Read the model definition and answer for the solid it produces. Units are mm, in the model's axes. Face numbers are marked on the shaded views. Round coordinates to 2 decimals unless told otherwise and drop trailing zeros. Write each loop counter-clockwise with the first axis right and the second up, starting at its lowest first coordinate (ties: lowest second). Pieces come first, ordered by that corner, then holes. Notation, with made-up numbers: (24, -15) -> (53, -15) arc R15 cw to (53, 1) -> close; hole circle Ø8 at (59.25, 41). An arc over 180 degrees is marked (long way). Return JSON: item names as keys, results as strings.
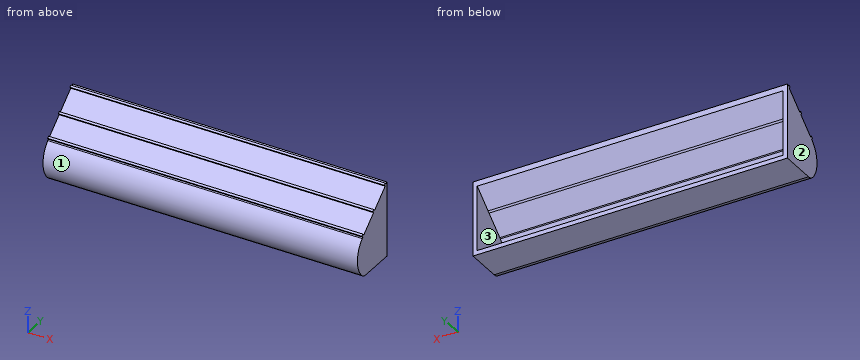
from build123d import *

# Parameters (mm, degrees)
F1_DEPTH    = 55.5
F2_DEPTH    = 297.5
F3_T        = 4
F3_T3_DEPTH = 305.5
F4_R        = 9
F5_R        = 9


# Not quite as in the source:
# - a shell that OpenCascade refuses in one call is made with other operations: the cavity is built on its own and cut out
# - a feature names something its author has since deleted; it is built from what else it names


with BuildPart() as f1:
    # F0 (on Right) → F1 (new body)
    with BuildSketch(Plane.YZ):
        with BuildLine():
            Line((-572.7275457045, -8.2819332473), (-535.7275457045, -8.2819332473))
            Line((-535.7275457045, -8.2819332473), (-535.7275457045, 62.5302098664))
            Line((-535.7275457045, 62.5302098664), (-537.1212494235, 61.363881769))
            Line((-537.1212494235, 61.363881769), (-538.6550321213, 60.0803278606))
            Line((-538.6550321213, 60.0803278606), (-555.619452014, 45.8835661626))
            Line((-555.619452014, 45.8835661626), (-557.1532347119, 44.6000122542))
            Line((-557.1532347119, 44.6000122542), (-572.8000965488, 31.5058557652))
            Line((-572.8000965488, 31.5058557652), (-574.3338792466, 30.2223018568))
            Line((-574.3338792466, 30.2223018568), (-575.2947741996, 29.4181719927))
            ThreePointArc((-575.2947741996, 29.4181719927), (-582.8883712939, 9.9636162879), (-572.7275457045, -8.2819332473))
        make_face()
        Polygon((-538.6550321213, 60.0803278606), (-537.1212494235, 61.363881769), (-538.404803332, 62.8976644668), (-539.9385860298, 61.6141105584), align=None)
        Polygon((-575.6174331551, 31.7560845546), (-574.3338792466, 30.2223018568), (-572.8000965488, 31.5058557652), (-574.0836504573, 33.0396384631), align=None)
        Polygon((-557.1532347119, 44.6000122542), (-555.619452014, 45.8835661626), (-556.9030059225, 47.4173488605), (-558.4367886203, 46.133794952), align=None)
    extrude(amount=F1_DEPTH)

    # F0 (on Right) → F2 (join)
    with BuildSketch(Plane.YZ):
        with BuildLine():
            Line((-572.7275457045, -8.2819332473), (-535.7275457045, -8.2819332473))
            Line((-535.7275457045, -8.2819332473), (-535.7275457045, 62.5302098664))
            Line((-535.7275457045, 62.5302098664), (-537.1212494235, 61.363881769))
            Line((-537.1212494235, 61.363881769), (-538.6550321213, 60.0803278606))
            Line((-538.6550321213, 60.0803278606), (-555.619452014, 45.8835661626))
            Line((-555.619452014, 45.8835661626), (-557.1532347119, 44.6000122542))
            Line((-557.1532347119, 44.6000122542), (-572.8000965488, 31.5058557652))
            Line((-572.8000965488, 31.5058557652), (-574.3338792466, 30.2223018568))
            Line((-574.3338792466, 30.2223018568), (-575.2947741996, 29.4181719927))
            ThreePointArc((-575.2947741996, 29.4181719927), (-582.8883712939, 9.9636162879), (-572.7275457045, -8.2819332473))
        make_face()
        Polygon((-538.6550321213, 60.0803278606), (-537.1212494235, 61.363881769), (-538.404803332, 62.8976644668), (-539.9385860298, 61.6141105584), align=None)
        Polygon((-575.6174331551, 31.7560845546), (-574.3338792466, 30.2223018568), (-572.8000965488, 31.5058557652), (-574.0836504573, 33.0396384631), align=None)
        Polygon((-557.1532347119, 44.6000122542), (-555.619452014, 45.8835661626), (-556.9030059225, 47.4173488605), (-558.4367886203, 46.133794952), align=None)
    extrude(amount=F2_DEPTH)

    # F3: shell of thickness 4, made by hand


with BuildPart() as f3_core1:
    # F3_t2: copy of F1
    add(f1.part)

    # the walls: a layer under each face that stays
    f3_faces = [f3_core1.faces().sort_by_distance(p)[0] for p in [
        (148.75, -582.8883712939, 9.9636162879),
        (0, -559.3362720247, 27.3078656098),
        (148.75, -574.9756562009, 30.9891932057),
        (148.75, -574.8505418062, 32.3978615088),
        (148.75, -573.441873503, 32.2727471141),
        (148.75, -564.9766656303, 38.0529340097),
        (148.75, -557.7950116661, 45.3669036031),
        (148.75, -557.6698972714, 46.7755719063),
        (148.75, -556.2612289683, 46.6504575116),
        (148.75, -547.1372420677, 52.9819470116),
        (148.75, -539.2968090756, 60.8472192095),
        (148.75, -539.1716946809, 62.2558875126),
        (148.75, -537.7630263777, 62.1307731179),
        (148.75, -536.424397564, 61.9470458177),
        (148.75, -554.2275457045, -8.2819332473),
        (297.5, -559.3362720247, 27.3078656098),
        (148.75, -574.8143267231, 29.8202369247),
    ]]
    thicken(f3_faces, amount=-F3_T, mode=Mode.SUBTRACT)

    # F3_s4 → F3_t3 (cut)
    with BuildSketch(Plane.YZ.offset(-4)):
        Polygon((-574.3902259788, 30.2273064326), (-571.266313851, 32.7894096737), (-568.6992060341, 29.721844278), (-571.7667714298, 27.1547364611), align=None)
        Polygon((-572.795091973, 31.5622024973), (-575.8676619445, 28.9387479484), (-573.3005541276, 25.8711825527), (-570.232988732, 28.4382903696), align=None)
        Polygon((-557.209581444, 44.60501683), (-554.586126895, 41.5324468586), (-551.5185614994, 44.0995546754), (-554.0856693162, 47.1671200711), align=None)
        Polygon((-555.6144474383, 45.9399128948), (-558.6870174097, 43.3164583458), (-556.1199095928, 40.2488929501), (-553.0523441972, 42.816000767), align=None)
        Polygon((-538.7113788535, 60.0853324364), (-536.0879243045, 57.0127624649), (-533.0203589088, 59.5798702818), (-535.5874667257, 62.6474356775), align=None)
        Polygon((-537.1162448477, 61.4202285011), (-540.1888148192, 58.7967739522), (-537.6217070023, 55.7292085565), (-534.5541416067, 58.2963163734), align=None)
    extrude(amount=F3_T3_DEPTH, mode=Mode.SUBTRACT)


with BuildPart() as f1_1:
    add(f1.part)

    # what is left inside the walls is the cavity
    f3_cavity = [f3_core1.part.solids().sort_by_distance(p)[0] for p in [
        (197, -535.767546, 26.516207),
    ]]
    add(f3_cavity, mode=Mode.SUBTRACT)

    # F4
    f4_edges = [f1_1.edges().sort_by_distance(p)[0] for p in [
        (148.75, -572.727546, -8.281933),
    ]]
    fillet(f4_edges, radius=F4_R)

    # F5
    f5_edges = [f1_1.edges().sort_by_distance(p)[0] for p in [
        (148.75, -571.376781, -4.281933),
    ]]
    fillet(f5_edges, radius=F5_R)


solid = f1_1.part
Item 1: For a pull along X with two mould halves and no side action, classify the marked faces 1, 2 and 3 as released by +X, released by -X, zero draft, split by the parting line, or undercut.
Worked answers:
{"face 1": "zero draft", "face 2": "released by -X", "face 3": "undercut"}
Item 2: Straight lines are drawn through the part: L1, parallel to X at y = -554.5, z = 26; L2, parallel to Z at x = 172.5, y = -571.5; L3, parallel to Z at x = 146, y = -552.5. For each, find the intervals that lie inside material, in ascending order. Write a range as [from, to].
Worked answers:
{"L1": "x = [0, 4], [293.5, 297.5]", "L2": "z = [-8.05, -3.41], [27.38, 32.59]", "L3": "z = [-8.28, -4.28], [43.28, 48.49]"}
Item 3: Section D-D (y = -548.5) is taken. Give the vertices of the cut face in (x, z).
Worked answers:
{"outline": "(0, -8.28) -> (297.5, -8.28) -> (297.5, 51.84) -> (0, 51.84) -> close; hole (4, -4.28) -> (293.5, -4.28) -> (293.5, 46.63) -> (4, 46.63) -> close"}
Item 4: Section A-A (x = 179) is taken. Give the vertices of the cut face in (y, z).
Worked answers:
{"outline": "(-575.85, -5.61) arc R9 ccw to (-569.46, -8.28) -> (-535.73, -8.28) -> (-535.73, -4.28) -> (-567.64, -4.28) arc R9 cw to (-574.84, -0.69) arc R20.51 cw to (-572.63, 26.43) -> (-535.73, 57.31) -> (-535.73, 62.53) -> (-537.12, 61.36) -> (-538.4, 62.9) -> (-539.94, 61.61) -> (-538.66, 60.08) -> (-555.62, 45.88) -> (-556.9, 47.42) -> (-558.44, 46.13) -> (-557.15, 44.6) -> (-572.8, 31.51) -> (-574.08, 33.04) -> (-575.62, 31.76) -> (-574.33, 30.22) -> (-575.29, 29.42) arc R24.51 ccw to start"}
Item 5: Section B-B (y = -562.5) is taken. Give the vertices of the cut face in (x, z), then the cut area to 3 significant figures.
Worked answers:
{"outline": "(0, -8.28) -> (297.5, -8.28) -> (297.5, 40.13) -> (0, 40.13) -> close; hole (4, -4.28) -> (293.5, -4.28) -> (293.5, 34.91) -> (4, 34.91) -> close", "area": "3,060 mm2"}
Item 6: Section C-C (z = 37.5) is taken. Give the vertices of the cut face in (x, y), then the cut area to 3 significant figures.
Worked answers:
{"outline": "(0, -565.64) -> (297.5, -565.64) -> (297.5, -535.73) -> (293.5, -535.73) -> (293.5, -559.4) -> (4, -559.4) -> (4, -535.73) -> (0, -535.73) -> close", "area": "2,040 mm2"}
Item 7: Flat-ended cylindrical pins translate along their axes: pin 1 (10 mm diameter, centred on x = 251, z = 43.5, fed in from -Y); pin 2 (12 mm diameter, centred on x = 48.5, z = 37, fed in from +Y); pin 3 (4 mm diameter, centred on x = 144.5, z = 50, fed in from -Y). Find the tip coordinate at first contact, or state that the pin passes through.
Worked answers:
{"pin 1": "stops at y = -564.44", "pin 2": "stops at y = -552.83", "pin 3": "stops at y = -553.09"}
